Geometry check sheet. Reference: the model listing, model coordinates, mm. A direction names the side the tool comes from. Give positions to 0.01 mm unless a question says otherwise; leave off trailing zeros. Write each loop counter-clockwise with the first axis right and the second up, starting at its lowest first coordinate (ties: lowest second). Pieces come first, ordered by that corner, then holes.
(1) Depth check by flat-ended pin: P1, Ø1.8, axis at x = -7.5, y = 5, coming from the +Z side. Enter the tip coordinate at first touch or a pass-through.
(2) Tool access check on faces 4 (the flat face through (0, -10, 2)), 5 (the flat face through (10.5, 7, 2)). Record the directions out of +Z, -Z, +X, -X, +Y, -Y that give a thin tool (end or side, any length) a straight path to the whole face; none if there is none.
(3) Cross-section at D-D (z = 1.65). Record the boundary of the cut face in (x, y).
(4) Cross-section at A-A (x = -7.5). Record the boundary of the cut face in (y, z).
(5) Cross-section at C-C (y = 8.5). Record the boundary of the cut face in (x, z), and give its area (3 significant figures).
(6) Thickness scan on line 1 along Y through (x, z) = (-7.5, 2.4); line 2 along X through (y, z) = (22.5, 1.45); line 3 along Y through (x, z) = (8.5, 2.4). Record the ranges inside material, lowest first.
(7) Cross-section at B-B (y = -5). Record the boundary of the cut face in (x, z), and give its area (3 significant figures).
(8) Mould release check, pull along X, two halves, no side actions. Record for faces 1 (the flat face through (0, 28, 2)), 2 (the flat face through (-10.5, 7, 2)), 3 (the cylindrical face through (6.39, -3.99, 1.97)): +X half, -X half, draft (parallel to the pull), parting line (faces both ways), or undercut.
```python
from build123d import *

# Parameters (mm, degrees)
SKETCH_1_R          = 1.5
EXTRUDE_1_DEPTH     = 4
FILLET_1_R          = 2
SKETCH_3_W          = 25.138692766
SKETCH_3_H          = 29.703861026
CUT_EXTRUDE_1_DEPTH = 38.446628687
SKETCH_4_W          = 21
SKETCH_4_H          = 14
EXTRUDE_2_DEPTH     = 4
SKETCH_5_W          = 7
SKETCH_5_H          = 34
CUT_EXTRUDE_2_DEPTH = 31.170349683


with BuildPart() as part:
    # 草图1 → 凸台-拉伸1 (new body)
    with BuildSketch(Plane.XY):
        Polygon((-10.5, 14), (10.5, 14), (10.5, 4), (34.5, 4), (34.5, -4), (10.5, -4), (10.5, -14), (-10.5, -14), align=None)
        with Locations((-7.5, 5)):
            Circle(SKETCH_1_R, mode=Mode.SUBTRACT)
        with Locations((7.5, 5)):
            Circle(SKETCH_1_R, mode=Mode.SUBTRACT)
        with Locations((-7.5, -5)):
            Circle(SKETCH_1_R, mode=Mode.SUBTRACT)
        with Locations((7.5, -5)):
            Circle(SKETCH_1_R, mode=Mode.SUBTRACT)
        with Locations((16.5, 0)):
            Circle(SKETCH_1_R, mode=Mode.SUBTRACT)
        with Locations((31.5, 0)):
            Circle(SKETCH_1_R, mode=Mode.SUBTRACT)
    extrude(amount=EXTRUDE_1_DEPTH)

    # 圆角1
    fillet_1_edges = [part.edges().sort_by_distance(p)[0] for p in [
        (10.5, 4, 2),
        (10.5, -4, 2),
    ]]
    fillet(fillet_1_edges, radius=FILLET_1_R)

    # 草图3 → 切除-拉伸1 (cut, through all)
    with BuildSketch(Plane.XY.offset(4)):
        with Locations((23.069346383, -0.851930513)):
            Rectangle(SKETCH_3_W, SKETCH_3_H)
    extrude(amount=-CUT_EXTRUDE_1_DEPTH, mode=Mode.SUBTRACT)

    # 草图4 → 凸台-拉伸2 (add)
    with BuildSketch(Plane.XY.offset(4)):
        with Locations((0, 21)):
            Rectangle(SKETCH_4_W, SKETCH_4_H)
    extrude(amount=-EXTRUDE_2_DEPTH)

    # 草图5 → 切除-拉伸2 (cut, through all)
    with BuildSketch(Plane.XY.offset(4)):
        with Locations((0, 7)):
            Rectangle(SKETCH_5_W, SKETCH_5_H)
    extrude(amount=-CUT_EXTRUDE_2_DEPTH, mode=Mode.SUBTRACT)


solid = part.part
```
Reply:
1. P1: passes through
2. face 4: +Z, -Z
2. face 5: +Z, -Z, +X, +Y, -Y
3. outline: (-10.5, -14) - (10.5, -14) - (10.5, 28) - (-10.5, 28) - close; hole circle Ø3 at (-7.5, -5); hole circle Ø3 at (-7.5, 5); hole (-3.5, -10) - (3.5, -10) - (3.5, 24) - (-3.5, 24) - close; hole circle Ø3 at (7.5, -5); hole circle Ø3 at (7.5, 5)
4. outline: (-14, 0) - (-6.5, 0) - (-6.5, 4) - (-14, 4) - close; (-3.5, 0) - (3.5, 0) - (3.5, 4) - (-3.5, 4) - close; (6.5, 0) - (28, 0) - (28, 4) - (6.5, 4) - close
5. outline: (-10.5, 0) - (-3.5, 0) - (-3.5, 4) - (-10.5, 4) - close; (3.5, 0) - (10.5, 0) - (10.5, 4) - (3.5, 4) - close
5. area: 56.0 mm2
6. line 1: y = -14 to -6.5, -3.5 to 3.5, 6.5 to 28
6. line 2: x = -10.5 to -3.5, 3.5 to 10.5
6. line 3: y = -14 to -6.12, -3.88 to 3.88, 6.12 to 28
7. outline: (-10.5, 0) - (-9, 0) - (-9, 4) - (-10.5, 4) - close; (-6, 0) - (-3.5, 0) - (-3.5, 4) - (-6, 4) - close; (3.5, 0) - (6, 0) - (6, 4) - (3.5, 4) - close; (9, 0) - (10.5, 0) - (10.5, 4) - (9, 4) - close
7. area: 32.0 mm2
8. face 1: draft
8. face 2: -X half
8. face 3: undercut
